from build123d import *

# Parameters (mm, degrees)
SKETCH3_W           = 27
SKETCH3_H           = 28
BOSS_EXTRUDE1_DEPTH = 2
SKETCH2_R           = 0.9
CUT_EXTRUDE1_DEPTH  = 10


with BuildPart() as part:
    # Sketch3 → Boss-Extrude1 (new body)
    with BuildSketch(Plane(origin=(0, 0, 0), x_dir=(1, 0, 0), z_dir=(0, 1, 0))):
        with Locations((0, -14)):
            Rectangle(SKETCH3_W, SKETCH3_H)
    extrude(amount=-BOSS_EXTRUDE1_DEPTH)

    # Sketch2 → Cut-Extrude1 (cut)
    with BuildSketch(Plane(origin=(0, 0, 0), x_dir=(1, 0, 0), z_dir=(0, 1, 0))):
        with Locations(Location((-10.5, -2, 0), (0, 0, 270))):
            Circle(SKETCH2_R)
        with Locations(Location((-10.5, -14.5, 0), (0, 0, 270))):
            Circle(SKETCH2_R)
        with Locations(Location((10.5, -14.5, 0), (0, 0, 270))):
            Circle(SKETCH2_R)
        with Locations(Location((10.5, -2, 0), (0, 0, 270))):
            Circle(SKETCH2_R)
    extrude(amount=-CUT_EXTRUDE1_DEPTH, mode=Mode.SUBTRACT)


solid = part.part
Build history of the part. All positions in model axes, mm. Coordinates: 2 decimals unless noted, no trailing zeros. Write each loop counter-clockwise with the first axis right and the second up, starting at its lowest first coordinate (ties: lowest second). Pieces come first, ordered by that corner, then holes.
(1) Cut at B-B on z = 2. List the corners of the cut face in (x, y).
(2) Drill centre lines: line 1 (X direction, y = -1.05, z = 14.5); line 2 (Z direction, x = 10.25, y = -0.75). Where is each one in solid material? Low to high.
(3) Mould opens along Z. For faces 1 (the cylindrical face through (-9.74, -0.99, 2.48)), 2 (the flat face through (0, -1, 0)), 3 (the flat face through (0, 0, 14)) say: pulls with the +Z half, pulls with the -Z half, needs draft (parallel to the pull), parting line crosses it, or undercut.
(4) Cut at A-A on x = -10.5. List the corners of the cut face in (y, z), and give its area (3 significant figures).
Working result:
1. outline: (-13.5, -2) - (-11.4, -2) - (-11.4, 0) - (-13.5, 0) - close; (-9.6, -2) - (9.6, -2) - (9.6, 0) - (-9.6, 0) - close; (11.4, -2) - (13.5, -2) - (13.5, 0) - (11.4, 0) - close
2. line 1: x = -13.5 to -11.4, -9.6 to 9.6, 11.4 to 13.5
2. line 2: z = 0 to 1.14, 2.86 to 13.64, 15.36 to 28
3. face 1: undercut
3. face 2: pulls with the -Z half
3. face 3: needs draft
4. outline: (-2, 0) - (0, 0) - (0, 1.1) - (-2, 1.1) - close; (-2, 2.9) - (0, 2.9) - (0, 13.6) - (-2, 13.6) - close; (-2, 15.4) - (0, 15.4) - (0, 28) - (-2, 28) - close
4. area: 48.8 mm2
